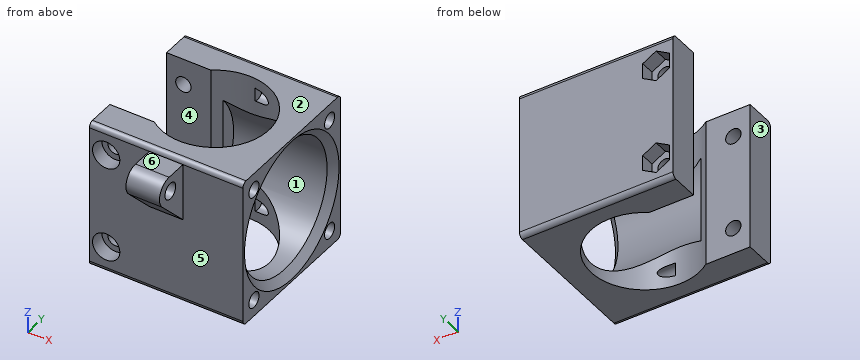
```python
from build123d import *

# Parameters (mm, degrees)
SKETCH1_W           = 31
SKETCH1_H           = 31
BOSS_EXTRUDE1_DEPTH = 16
FILLET1_R           = 1
SKETCH2_R           = 13.5
CUT_EXTRUDE1_DEPTH  = 21
SKETCH3_R           = 1.6
CUT_EXTRUDE2_DEPTH  = 15
CUT_EXTRUDE3_DEPTH  = 39.173943993
SKETCH5_R           = 1.6
CUT_EXTRUDE4_DEPTH  = 47.669047659
CUT_EXTRUDE5_DEPTH  = 2.95
SKETCH7_R           = 2.85
CUT_EXTRUDE6_DEPTH  = 2.95
BOSS_EXTRUDE2_START = -12.5
BOSS_EXTRUDE2_DEPTH = 7
SKETCH9_R           = 1.70000037
CUT_EXTRUDE7_DEPTH  = 44.213437626
CHAMFER1_SIZE       = 1.5


with BuildPart() as part:
    # Sketch1 → Boss-Extrude1 (new, symmetric)
    with BuildSketch(Plane(origin=(0, 0, 0), x_dir=(0, 0, -1), z_dir=(1, 0, 0))):
        with Locations((-15.5, 0)):
            Rectangle(SKETCH1_W, SKETCH1_H)
    extrude(amount=BOSS_EXTRUDE1_DEPTH, both=True)

    # Fillet1
    fillet1_edges = [part.edges().sort_by_distance(p)[0] for p in [
        (0, -15.5, 0),
        (0, -15.5, 31),
        (0, 15.5, 31),
        (0, 15.5, 0),
    ]]
    fillet(fillet1_edges, radius=FILLET1_R)

    # Sketch2 → Cut-Extrude1 (cut)
    with BuildSketch(Plane(origin=(16, 0, 0), x_dir=(0, 0, -1), z_dir=(1, 0, 0))):
        with Locations((-15.5, 0)):
            Circle(SKETCH2_R)
    extrude(amount=-CUT_EXTRUDE1_DEPTH, mode=Mode.SUBTRACT)

    # Sketch3 → Cut-Extrude2 (cut)
    with BuildSketch(Plane(origin=(16, 0, 0), x_dir=(0, 0, -1), z_dir=(1, 0, 0))):
        with Locations((-27.5, 12)):
            Circle(SKETCH3_R)
        with Locations((-3.5, 12)):
            Circle(SKETCH3_R)
        with Locations((-3.5, -12)):
            Circle(SKETCH3_R)
        with Locations((-27.5, -12)):
            Circle(SKETCH3_R)
    extrude(amount=-CUT_EXTRUDE2_DEPTH, mode=Mode.SUBTRACT)

    # Sketch4 → Cut-Extrude3 (cut, through all)
    with BuildSketch(Plane.XY.offset(31)):
        with BuildLine():
            Line((-6.75, 9), (-16, 9))
            Line((-16, 9), (-16, -9))
            Line((-16, -9), (-6.75, -9))
            ThreePointArc((-6.75, -9), (11.25, 0), (-6.75, 9))
        make_face()
    extrude(amount=-CUT_EXTRUDE3_DEPTH, mode=Mode.SUBTRACT)

    # Sketch5 → Cut-Extrude4 (cut, through all)
    with BuildSketch(Plane(origin=(0, 15.5, 0), x_dir=(1, 0, 0), z_dir=(0, 1, 0))):
        with Locations(Location((-12.5, -5.5, 0), (0, 0, 270))):
            Circle(SKETCH5_R)
        with Locations(Location((-12.5, -25.5, 0), (0, 0, 270))):
            Circle(SKETCH5_R)
    extrude(amount=-CUT_EXTRUDE4_DEPTH, mode=Mode.SUBTRACT)

    # Sketch6 → Cut-Extrude5 (cut)
    with BuildSketch(Plane(origin=(0, 15.5, 0), x_dir=(1, 0, 0), z_dir=(0, 1, 0))):
        Polygon((-12.5, -8.725425014), (-9.7067, -7.112712507), (-9.7067, -3.887287493), (-12.5, -2.274574986), (-15.2933, -3.887287493), (-15.2933, -7.112712507), align=None)
        Polygon((-9.7067, -27.112712507), (-9.7067, -23.887287493), (-12.5, -22.274574986), (-15.2933, -23.887287493), (-15.2933, -27.112712507), (-12.5, -28.725425014), align=None)
    extrude(amount=-CUT_EXTRUDE5_DEPTH, mode=Mode.SUBTRACT)

    # Sketch7 → Cut-Extrude6 (cut)
    with BuildSketch(Plane.XZ.offset(15.5)):
        with Locations(Location((-12.5, 25.5, 0), (0, 0, 270))):
            Circle(SKETCH7_R)
        with Locations(Location((-12.5, 5.5, 0), (0, 0, 270))):
            Circle(SKETCH7_R)
    extrude(amount=-CUT_EXTRUDE6_DEPTH, mode=Mode.SUBTRACT)

    # Sketch8 → Boss-Extrude2 (add)
    with BuildSketch(Plane(origin=(16, 0, 0), x_dir=(0, 0, -1), z_dir=(1, 0, 0)).offset(BOSS_EXTRUDE2_START)):
        with BuildLine():
            Line((-30, -15.5), (-30, -19.893951988))
            ThreePointArc((-30, -19.893951988), (-28.14780731, -22.694961806), (-24.845223874, -22.087329999))
            Line((-24.845223874, -22.087329999), (-18, -15.5))
            Line((-18, -15.5), (-30, -15.5))
        make_face()
    extrude(amount=-BOSS_EXTRUDE2_DEPTH)

    # Sketch9 → Cut-Extrude7 (cut, through all)
    with BuildSketch(Plane(origin=(3.5, 0, 0), x_dir=(0, 0, -1), z_dir=(1, 0, 0))):
        with Locations((-26.749999873, -19.500000979)):
            Circle(SKETCH9_R)
    extrude(amount=-CUT_EXTRUDE7_DEPTH, mode=Mode.SUBTRACT)

    # Chamfer1
    chamfer1_edges = [part.edges().sort_by_distance(p)[0] for p in [
        (16, 0, 29),
    ]]
    chamfer(chamfer1_edges, length=CHAMFER1_SIZE)


solid = part.part
```
CAD build for the part. Positions are in the model's coordinates, mm. Face numbers are marked on the shaded views. A direction names the side the tool comes from. Round coordinates to 2 decimals unless told otherwise and drop trailing zeros. Order: outer loops, then holes, each group sorted by start corner. A loop starts at its lowest first (then second) coordinate and runs counter-clockwise, first axis right, second up.
Item 1: Probe line 1 along X through (y, z) = (-14, 5); line 2 along Y through (x, z) = (-13.5, 10); line 3 along Y through (x, z) = (10, 27). List the from-to ranges inside material, lowest first.
Item 2: Saw through at B-B on z = 15.5. Write the cut outline in (x, y).
Item 3: Saw through at A-A on y = 0. Write the cut outline in (x, z), then the cut area to 4 significant figures.
Item 4: Saw through at D-D on x = 9. Write the cut outline in (y, z).
Item 5: Tool access for the marked faces 4, 5 and 6: list every direction of +Z, -Z, +X, -X, +Y, -Y with a clear straight run to the whole face (end or side of a thin tool).
Item 6: Pin check, flat tips, straight feed: pin 1 (1.9 mm diameter, centred on x = -12.5, z = 5.5, fed in from -Y); pin 2 (3.5 mm diameter, centred on x = -12.5, z = 25.5, fed in from +Y); pin 3 (6 mm diameter, centred on x = -9.5, z = 8.5, fed in from -Y); pin 4 (4 mm diameter, centred on y = -12.5, z = 18.5, fed in from +X). Stop position of each tip, or through.
Item 7: Saw through at C-C on x = -1.5. Write the cut outline in (y, z), then the cut area to 3 significant figures.
Item 8: Mould opens along Z. For the marked faces 1, 2 and 3 say: pulls with the +Z half, pulls with the -Z half, needs draft (parallel to the pull), parting line crosses it, or undercut.
Reported:
1. line 1: x = -16 to -15.31, -9.69 to 16
1. line 2: y = -15.5 to -9, 9 to 15.5
1. line 3: y = -15.5 to -13.52, -10.48 to -7.07, 7.07 to 10.48, 13.52 to 15.5
2. outline: (-16, -15.5) - (16, -15.5) - (16, -15) - (14.5, -13.5) - (-5, -13.5) - (-5, -10.08) arc R11.25 cw to (-6.75, -9) - (-16, -9) - close; (-16, 9) - (-6.75, 9) arc R11.25 cw to (-5, 10.08) - (-5, 13.5) - (14.5, 13.5) - (16, 15) - (16, 15.5) - (-16, 15.5) - close
3. outline: (11.25, 0) - (16, 0) - (16, 0.5) - (14.5, 2) - (11.25, 2) - close; (11.25, 29) - (14.5, 29) - (16, 30.5) - (16, 31) - (11.25, 31) - close
3. area: 16.75 mm2
4. outline: (-15.5, 1) arc R1 ccw to (-14.5, 0) - (-6.75, 0) - (-6.75, 3.81) arc R13.5 cw to (-6.75, 27.19) - (-6.75, 31) - (-14.5, 31) arc R1 ccw to (-15.5, 30) - close; (6.75, 0) - (14.5, 0) arc R1 ccw to (15.5, 1) - (15.5, 30) arc R1 ccw to (14.5, 31) - (6.75, 31) - (6.75, 27.19) arc R13.5 cw to (6.75, 3.81) - close; hole circle Ø3.2 at (-12, 3.5); hole circle Ø3.2 at (-12, 27.5); hole circle Ø3.2 at (12, 3.5); hole circle Ø3.2 at (12, 27.5)
5. face 4: +Z, -Z, -X
5. face 5: -Z, -Y
5. face 6: +Z, +X, -X, -Y
6. pin 1: passes through
6. pin 2: stops at y = 12.55
6. pin 3: stops at y = -15.5
6. pin 4: stops at x = 15.85
7. outline: (-22.09, 24.85) - (-15.5, 18) - (-15.5, 1) arc R1 ccw to (-14.5, 0) - (-11.15, 0) - (-11.15, 7.89) arc R13.5 cw to (-11.15, 23.11) - (-11.15, 31) - (-14.5, 31) arc R1 ccw to (-15.5, 30) - (-19.89, 30) arc R3.04 ccw to start; (11.15, 0) - (14.5, 0) arc R1 ccw to (15.5, 1) - (15.5, 30) arc R1 ccw to (14.5, 31) - (11.15, 31) - (11.15, 23.11) arc R13.5 cw to (11.15, 7.89) - close; hole circle Ø3.4 at (-19.5, 26.75)
7. area: 270 mm2
8. face 1: undercut
8. face 2: pulls with the +Z half
8. face 3: needs draft
